Part print with two shaded views. Sizes in mm from the minimum x, y, z corner. A direction names the side the tool comes from. Give positions to 0.01 mm unless a question says otherwise; leave off trailing zeros. Write each loop counter-clockwise with the first axis right and the second up, starting at its lowest first coordinate (ties: lowest second). Pieces come first, ordered by that corner, then holes.
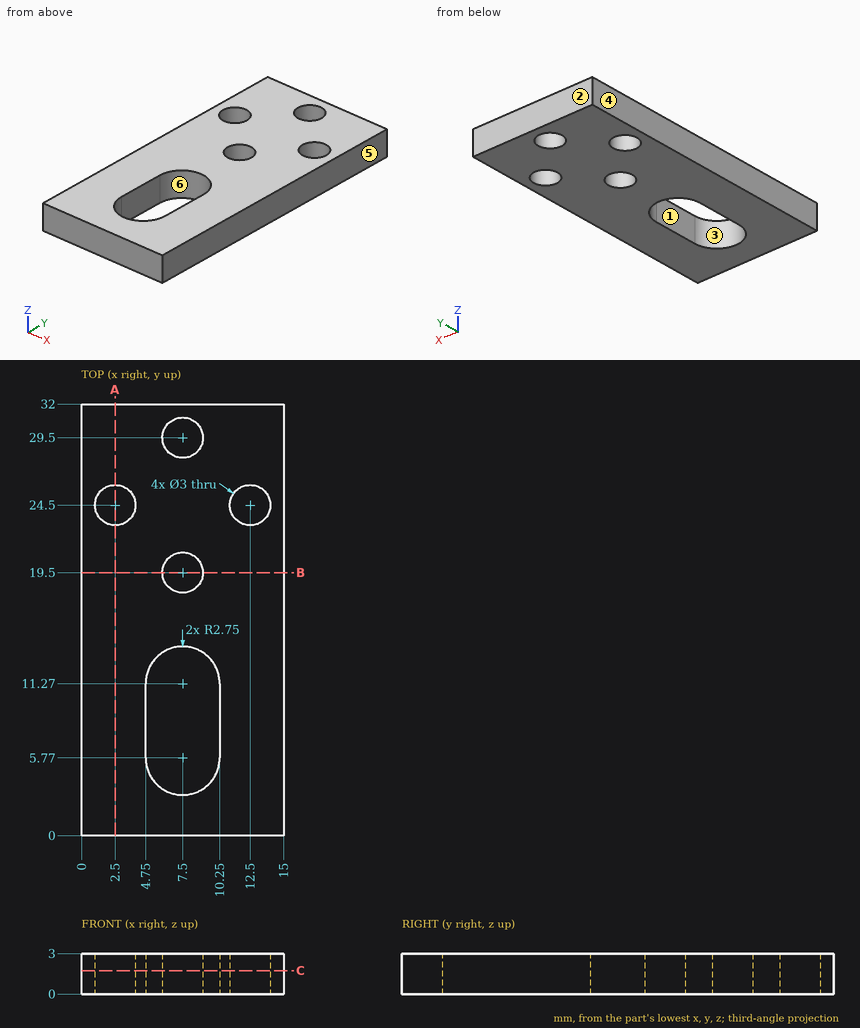
(1) 3-axis set-ups, long thin cutter, end or side, ignore diameter. For the marked faces 5 and 6: which of +Z, -Z, +X, -X, +Y, -Y reach the whole face in a straight line?
(2) Saw through at B-B, the plane y = 19.5. List the corners of the cut face in (x, z).
(3) Mould opens along Y. For the marked faces 1, 2, 3 and 4 say: +Y half, -Y half, draft (parallel to the pull), parting line (faces both ways), or undercut.
(4) Probe line 1 (Y direction, x = 7.5, z = 1.2); line 2 (X direction, y = 24.5, z = 2.25); line 3 (X direction, y = 10.5, z = 0.8). List the from-to ranges inside material, lowest first.
(5) Saw through at C-C, the plane z = 1.75. List the corners of the cut face in (x, y).
(6) Saw through at A-A, the plane x = 2.5. List the corners of the cut face in (y, z).
(7) Drop a flat-ended pin along its axis: pin 1 (1.8 mm diameter, centred on x = 7.5, y = 19.5, fed in from -Z). Give the stop position or say it passes through.
Computed values:
1. face 5: +Z, -Z, +X, +Y, -Y
1. face 6: +Z, -Z
2. outline: (0, 0) - (6, 0) - (6, 3) - (0, 3) - close; (9, 0) - (15, 0) - (15, 3) - (9, 3) - close
3. face 1: undercut
3. face 2: +Y half
3. face 3: undercut
3. face 4: draft
4. line 1: y = 0 to 3.02, 14.02 to 18, 21 to 28, 31 to 32
4. line 2: x = 0 to 1, 4 to 11, 14 to 15
4. line 3: x = 0 to 4.75, 10.25 to 15
5. outline: (0, 0) - (15, 0) - (15, 32) - (0, 32) - close; hole circle Ø3 at (2.5, 24.5); hole (4.75, 5.77) arc R2.75 ccw to (10.25, 5.77) - (10.25, 11.27) arc R2.75 ccw to (4.75, 11.27) - close; hole circle Ø3 at (7.5, 19.5); hole circle Ø3 at (7.5, 29.5); hole circle Ø3 at (12.5, 24.5)
6. outline: (0, 0) - (23, 0) - (23, 3) - (0, 3) - close; (26, 0) - (32, 0) - (32, 3) - (26, 3) - close
7. pin 1: passes through
